Work out the finished part from the listing and answer in its coordinate system (mm). Face numbers are marked on the shaded views. A direction names the side the tool comes from. Round coordinates to 2 decimals unless told otherwise and drop trailing zeros. Write each loop counter-clockwise with the first axis right and the second up, starting at its lowest first coordinate (ties: lowest second). Pieces come first, ordered by that corner, then holes.
1. Find section C-C (x = -1). Write down the section's boundary in (y, z).
2. Straight lines are drawn through the part: probe 1 along Y at (x, z) = (14.5, 5); probe 2 along Z at (x, y) = (-14, -19); probe 3 along Y at (x, z) = (-0.5, 2.5). For each, find the intervals that lie inside material, in ascending order.
3. Find section A-A (y = -4.5). Write down the section's boundary in (x, z), and give its area (3 significant figures).
4. A tool of negligible diameter and unlimited length cuts with its end or side. For the marked faces 1, 2 and 3, from which of +Z, -Z, +X, -X, +Y, -Y can it reach the whole face along a straight path? Write none if from no direction.
5. Flat-ended cylindrical pins translate along their axes: pin 1 Ø1.2 at (y, z) = (1, 18.5) entering from +X; pin 2 Ø5 at (x, y) = (0, 0) entering from -Z; pin 3 Ø23.5 at (y, z) = (0, 0) entering from -X; pin 4 Ø12 at (x, y) = (12.5, -8.5) entering from -Z. Find the tip coordinate at first contact, or state that the pin passes through.
6. Find section D-D (z = 19.25). Write down the section's boundary in (x, y).
7. Find section B-B (z = 8). Write down the section's boundary in (x, y), and give its area (3 significant figures).
8. Determine the mould class of the marked faces 4, 5 and 6 for opening direction Y: pulls with the +Y half, pulls with the -Y half, needs draft (parallel to the pull), parting line crosses it, or undercut.
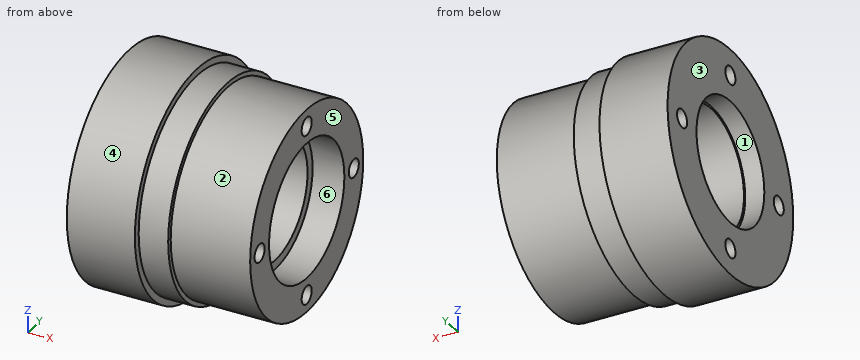
```python
from build123d import *

# Parameters (mm, degrees)
SKETCH2_R          = 2
CUT_EXTRUDE1_DEPTH = 10
SKETCH3_R          = 2
CUT_EXTRUDE2_DEPTH = 10


with BuildPart() as part:
    # Sketch1 → Revolve1 (revolve)
    with BuildSketch(Plane.XY, mode=Mode.PRIVATE) as revolve1_sk:
        Polygon((-19.5, 13.5), (-15.3, 13.5), (-15.3, 13), (12.5, 13), (12.5, 15), (19.5, 15), (19.5, 22.5), (2, 22.5), (2, 23.5), (-4.5, 23.5), (-4.5, 25), (-19.5, 25), align=None)
    revolve(revolve1_sk.sketch.rotate(Axis((-19.5, 0, 0), (1, 0, 0)), 180), axis=Axis((-19.5, 0, 0), (1, 0, 0)))

    # Sketch2 → Cut-Extrude1 (cut)
    with BuildSketch(Plane(origin=(19.5, 0, 0), x_dir=(0, 0, -1), z_dir=(1, 0, 0))):
        with Locations((0, 18.75)):
            Circle(SKETCH2_R)
        with Locations((18.75, 0)):
            Circle(SKETCH2_R)
        with Locations((0, -18.75)):
            Circle(SKETCH2_R)
        with Locations((-18.75, 0)):
            Circle(SKETCH2_R)
    extrude(amount=-CUT_EXTRUDE1_DEPTH, mode=Mode.SUBTRACT)

    # Sketch3 → Cut-Extrude2 (cut)
    with BuildSketch(Plane.ZY.offset(19.5)):
        with Locations((0, 19.25)):
            Circle(SKETCH3_R)
        with Locations((19.25, 0)):
            Circle(SKETCH3_R)
        with Locations((0, -19.25)):
            Circle(SKETCH3_R)
        with Locations((-19.25, 0)):
            Circle(SKETCH3_R)
    extrude(amount=-CUT_EXTRUDE2_DEPTH, mode=Mode.SUBTRACT)


solid = part.part
```
Worked answers:
1. outline: circle Ø47 at (0, 0); hole circle Ø26 at (0, 0)
2. probe 1: y = -21.94 to -14.14, 14.14 to 21.94
2. probe 2: z = -16.25 to -1.98, 1.98 to 16.25
2. probe 3: y = -23.37 to -12.76, 12.76 to 23.37
3. outline: (-19.5, -24.59) - (-4.5, -24.59) - (-4.5, -23.07) - (2, -23.07) - (2, -22.05) - (19.5, -22.05) - (19.5, -14.31) - (12.5, -14.31) - (12.5, -12.2) - (-15.3, -12.2) - (-15.3, -12.73) - (-19.5, -12.73) - close; (-19.5, 12.73) - (-15.3, 12.73) - (-15.3, 12.2) - (12.5, 12.2) - (12.5, 14.31) - (19.5, 14.31) - (19.5, 22.05) - (2, 22.05) - (2, 23.07) - (-4.5, 23.07) - (-4.5, 24.59) - (-19.5, 24.59) - close
3. area: 824 mm2
4. face 1: -X
4. face 2: +X
4. face 3: +Z, -Z, -X, +Y, -Y
5. pin 1: stops at x = 9.5
5. pin 2: stops at z = -23.5
5. pin 3: passes through
5. pin 4: stops at z = -22.36
6. outline: (-19.5, -15.95) - (-4.5, -15.95) - (-4.5, -13.48) - (2, -13.48) - (2, -11.65) - (19.5, -11.65) - (19.5, -1.94) - (9.5, -1.94) - (9.5, 1.94) - (19.5, 1.94) - (19.5, 11.65) - (2, 11.65) - (2, 13.48) - (-4.5, 13.48) - (-4.5, 15.95) - (-19.5, 15.95) - (-19.5, 2) - (-9.5, 2) - (-9.5, -2) - (-19.5, -2) - close
7. outline: (-19.5, -23.69) - (-4.5, -23.69) - (-4.5, -22.1) - (2, -22.1) - (2, -21.03) - (19.5, -21.03) - (19.5, -12.69) - (12.5, -12.69) - (12.5, -10.25) - (-15.3, -10.25) - (-15.3, -10.87) - (-19.5, -10.87) - close; (-19.5, 10.87) - (-15.3, 10.87) - (-15.3, 10.25) - (12.5, 10.25) - (12.5, 12.69) - (19.5, 12.69) - (19.5, 21.03) - (2, 21.03) - (2, 22.1) - (-4.5, 22.1) - (-4.5, 23.69) - (-19.5, 23.69) - close
7. area: 895 mm2
8. face 4: parting line crosses it
8. face 5: needs draft
8. face 6: undercut
